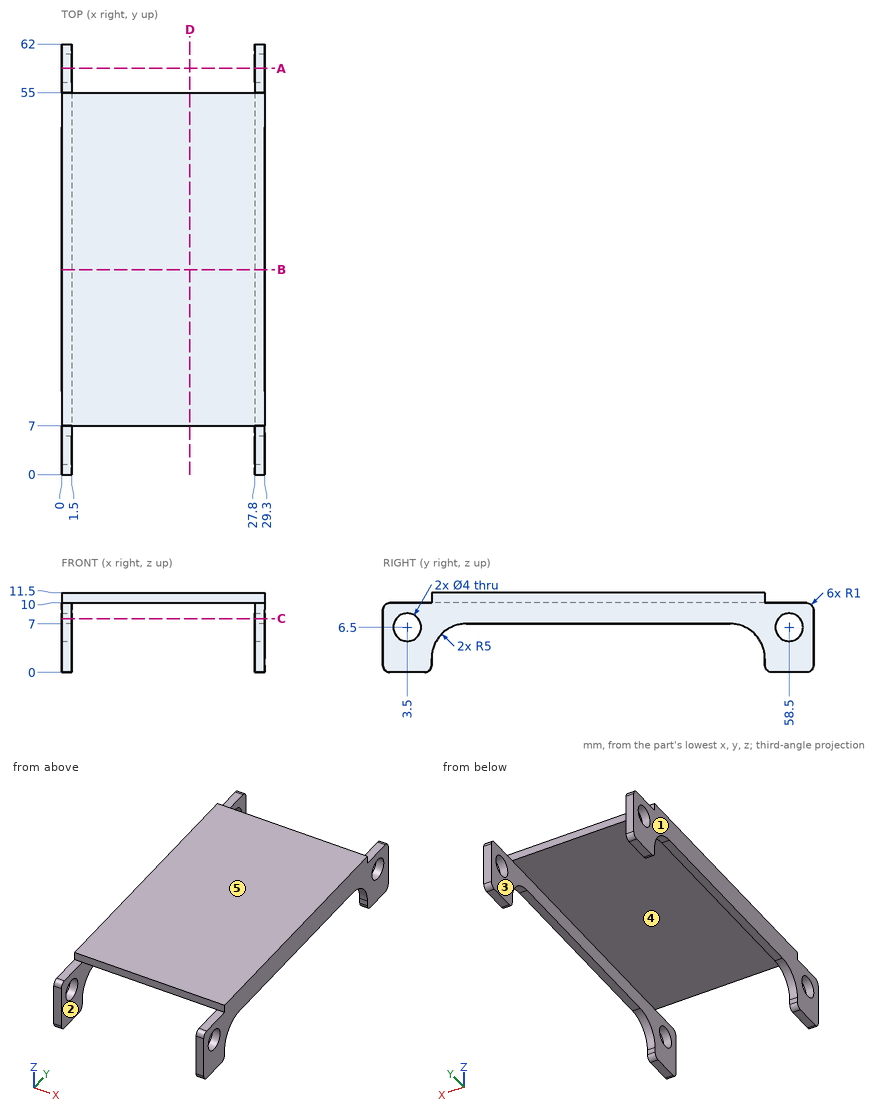
Geometry check sheet. Reference: drawing and pictorial views, mm from the part's lowest x, y, z. A direction names the side the tool comes from. Round coordinates to 2 decimals unless told otherwise and drop trailing zeros. Loops run counter-clockwise (first coordinate to the right, second up) from the corner with the lowest first, then second, coordinate; pieces in that order, holes last. Notation, with made-up numbers: (84, -32) - (91, -32) arc R17 cw to (91, -9) - close; hole circle Ø11 at (18, 74.5). An arc over 180 degrees is marked (long way). Answer in a Markdown table with one row per item. Add a question column.
Q1. Section check A-A on y = 58.5. Enter the section's corners in (x, z), plus the area to 3 significant figures.
Q2. Tool access check on the marked faces 1 and 2. Record the directions out of +Z, -Z, +X, -X, +Y, -Y that give a thin tool (end or side, any length) a straight path to the whole face; none if there is none.
Q3. Section check B-B on y = 29.5. Enter the section's corners in (x, z), plus the area to 4 significant figures.
Q4. Section check C-C on z = 7.75. Enter the section's corners in (x, y).
Q5. Gauge pin test, flat ends, axial feed: pin 1 (2.5 mm diameter, centred on y = 58.5, z = 6.5, fed in from +X); pin 2 (1 mm diameter, centred on x = 18, y = 35, fed in from -Z); pin 3 (0.8 mm diameter, centred on x = 1, y = 4.5, fed in from +Z); pin 4 (0.8 mm diameter, centred on x = 29, y = 39, fed in from -Z). Record the tip position at first contact, or that the pin passes through.
Q6. Material ranges on line 1 (Z direction, x = 0.85, y = 58.5); line 2 (X direction, y = 21.5, z = 8.25); line 3 (Z direction, x = 1.75, y = 53.5), recorded low to high.
Q7. Release check for a two-part mould opening along Z. For the marked faces 3, 4 and 5 record: pulls with the +Z half, pulls with the -Z half, needs draft (parallel to the pull), parting line crosses it, or undercut.
Q8. Section check D-D on x = 18.5. Enter the section's corners in (y, z), plus the area to 3 significant figures.
Found:
| question | item | result |
|---|---|---|
| 1 | outline | (0, 0) - (1.5, 0) - (1.5, 4.5) - (0, 4.5) - close; (0, 8.5) - (1.5, 8.5) - (1.5, 10) - (0, 10) - close; (27.8, 0) - (29.3, 0) - (29.3, 4.5) - (27.8, 4.5) - close; (27.8, 8.5) - (29.3, 8.5) - (29.3, 10) - (27.8, 10) - close |
| 1 | area | 18.0 mm² |
| 2 | face 1 | +Z, -Z, -X, +Y, -Y |
| 2 | face 2 | -Z, +Y, -Y |
| 3 | outline | (0, 7) - (1.5, 7) - (1.5, 10) - (27.8, 10) - (27.8, 7) - (29.3, 7) - (29.3, 11.5) - (0, 11.5) - close |
| 3 | area | 52.95 mm² |
| 4 | outline | (0, 0) - (1.5, 0) - (1.5, 1.94) - (0, 1.94) - close; (0, 5.06) - (1.5, 5.06) - (1.5, 56.94) - (0, 56.94) - close; (0, 60.06) - (1.5, 60.06) - (1.5, 62) - (0, 62) - close; (27.8, 0) - (29.3, 0) - (29.3, 1.94) - (27.8, 1.94) - close; (27.8, 5.06) - (29.3, 5.06) - (29.3, 56.94) - (27.8, 56.94) - close; (27.8, 60.06) - (29.3, 60.06) - (29.3, 62) - (27.8, 62) - close |
| 5 | pin 1 | passes through |
| 5 | pin 2 | stops at z = 10 |
| 5 | pin 3 | stops at z = 10 |
| 5 | pin 4 | stops at z = 7 |
| 6 | line 1 | z = 0 to 4.5, 8.5 to 10 |
| 6 | line 2 | x = 0 to 1.5, 27.8 to 29.3 |
| 6 | line 3 | z = 10 to 11.5 |
| 7 | face 3 | needs draft |
| 7 | face 4 | pulls with the -Z half |
| 7 | face 5 | pulls with the +Z half |
| 8 | outline | (7, 10) - (55, 10) - (55, 11.5) - (7, 11.5) - close |
| 8 | area | 72.0 mm² |
